from build123d import *

# Parameters (mm, degrees)
SALIENTE_EXTRUIR1_DEPTH = 25
CROQUIS2_W              = 100
CROQUIS2_H              = 25
SALIENTE_EXTRUIR2_DEPTH = 50
CROQUIS3_R              = 8.912899487
SALIENTE_EXTRUIR3_DEPTH = 10


with BuildPart() as part:
    # Croquis1 → Saliente-Extruir1 (new body)
    with BuildSketch(Plane(origin=(0, 0, 0), x_dir=(1, 0, 0), z_dir=(0, 1, 0))):
        with BuildLine():
            Line((-50, 0), (50, 0))
            ThreePointArc((50, 0), (26.377279403, 21.486732346), (12, 50))
            Line((12, 50), (-12, 50))
            ThreePointArc((-12, 50), (-26.377279403, 21.486732346), (-50, 0))
        make_face()
    extrude(amount=SALIENTE_EXTRUIR1_DEPTH)

    # Croquis2 → Saliente-Extruir2 (add)
    with BuildSketch(Plane.XY):
        with Locations((0, 12.5)):
            Rectangle(CROQUIS2_W, CROQUIS2_H)
    extrude(amount=SALIENTE_EXTRUIR2_DEPTH)

    # Croquis3 → Saliente-Extruir3 (add)
    with BuildSketch(Plane(origin=(50, 0, 0), x_dir=(0, 0, -1), z_dir=(1, 0, 0))):
        with Locations((-25, 12.5)):
            Circle(CROQUIS3_R)
    saliente_extruir3 = extrude(amount=SALIENTE_EXTRUIR3_DEPTH)

    # Simetría1: Saliente-Extruir3 across plane
    add(saliente_extruir3.mirror(Plane(origin=(0, 0, 0), x_dir=(0, 0, 1), z_dir=(1, 0, 0))))


solid = part.part
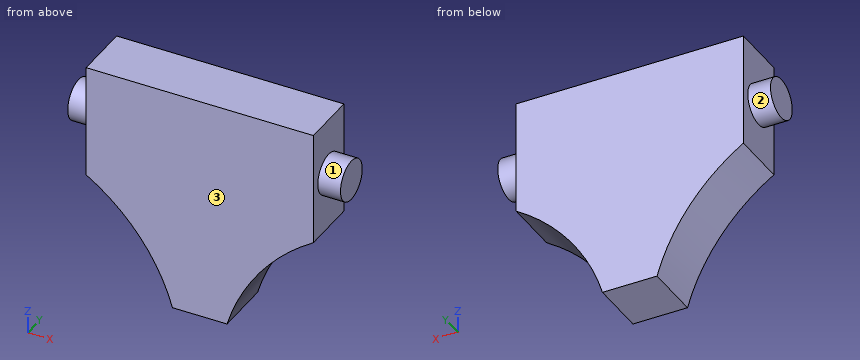
Geometry: final body of the model. Coordinates: model frame, mm. Face numbers are marked on the shaded views. A direction names the side the tool comes from. Give positions to 0.01 mm unless a question says otherwise; leave off trailing zeros. Loops run counter-clockwise (first coordinate to the right, second up) from the corner with the lowest first, then second, coordinate; pieces in that order, holes last. Notation, with made-up numbers: (-18, 29.5) - (40, 29.5) arc R25 ccw to (40, 51.5) - close; hole circle Ø7 at (74, 75.5). An arc over 180 degrees is marked (long way). One line per question, with ' | ' between items. Start each with the question number.
(1) Section query C-C on x = 32. Return loops of the section in (y, z), then the cut area to 3 significant figures.
(2) Contact query for flat-ended pins moving along their axis: pin 1 (4 mm diameter, centred on x = -39.5, y = 9.5, fed in from -Z); pin 2 (12 mm diameter, centred on x = 25, y = 19, fed in from -Z); pin 3 (6 mm diameter, centred on y = 7, z = -12.5, fed in from -X). Output: stop coordinate, or through.
(3) Section query A-A on y = 12.5. Return loops of the section in (x, z).
(4) Section query B-B on z = 25. Return loops of the section in (x, y).
(5) Reachability of the marked faces 1, 2 and 3 from +Z, -Z, +X, -X, +Y, -Y: full face, straight path, thin tool, end or side. Return the list, or none.
(6) Ray query, line 1 (X direction, y = 7.5, z = 5.5); line 2 (Z direction, x = 39.5, y = 14.5); line 3 (Z direction, x = 15, y = 23.25). Return the intervals inside material, ascending. Write a range as from..to.
(7) Section query D-D on x = -36. Return loops of the section in (y, z).
The answers:
1) outline: (0, -14.81) - (25, -14.81) - (25, 50) - (0, 50) - close | area: 1,620 mm2
2) pin 1: z = -9.39 | pin 2: z = -32.94 | pin 3: x = -37.38
3) outline: (-60, 16.09) - (-50, 16.09) - (-50, 0) arc R87.81 cw to (-12, -50) - (12, -50) arc R87.81 cw to (50, 0) - (50, 16.09) - (60, 16.09) - (60, 33.91) - (50, 33.91) - (50, 50) - (-50, 50) - (-50, 33.91) - (-60, 33.91) - close
4) outline: (-60, 3.59) - (-50, 3.59) - (-50, 0) - (50, 0) - (50, 3.59) - (60, 3.59) - (60, 21.41) - (50, 21.41) - (50, 25) - (-50, 25) - (-50, 21.41) - (-60, 21.41) - close
5) face 1: +X | face 2: -X | face 3: +Z, -Z, +X, -X, -Y
6) line 1: -50..50 | line 2: -7.64..50 | line 3: -41.41..50
7) outline: (0, -10.78) - (25, -10.78) - (25, 50) - (0, 50) - close
